```python
from build123d import *

# Parameters (mm, degrees)
F0_W     = 5
F0_H     = 3.3166247904
F0_H_2   = 16
F0_H_3   = 14.6833752096
F0_H_4   = 2
F1_DEPTH = 3
F2_DEPTH = 11
F3_START = 3
F3_DEPTH = 5
F4_R     = 3
F5_F1_R  = 1
F5_F2_R  = 0.9999


# Not quite as in the source:
# - a fillet or chamfer is up to 0.001 mm smaller than in the source, because OpenCascade refuses the exact size


with BuildPart() as f1:
    # F0 (on Top) → F1 (new body)
    with BuildSketch(Plane.XY):
        Rectangle(F0_W, F0_H)
        with Locations((0, -26.3416876048)):
            Rectangle(F0_W, F0_H_2)
        with Locations((0, -11)):
            Rectangle(F0_W, F0_H_3)
        with Locations((0, -2.6583123952)):
            Rectangle(F0_W, F0_H_4)
        Polygon((2.5, -34.3416876048), (-2.5, -34.3416876048), (-2.5, -38.3416876048), (0, -38.3416876048), (2.5, -38.3416876048), align=None)
    extrude(amount=F1_DEPTH)

    # F0 (on Top) → F2 (join)
    with BuildSketch(Plane.XY):
        Rectangle(F0_W, F0_H)
        with Locations((0, -2.6583123952)):
            Rectangle(F0_W, F0_H_4)
        Polygon((2.5, -34.3416876048), (-2.5, -34.3416876048), (-2.5, -38.3416876048), (0, -38.3416876048), (2.5, -38.3416876048), align=None)
        with Locations((0, -26.3416876048)):
            Rectangle(F0_W, F0_H_2)
    extrude(amount=F2_DEPTH)

    # F0 (on Top) → F3 (cut)
    with BuildSketch(Plane.XY.offset(F3_START)):
        with Locations((0, -2.6583123952)):
            Rectangle(F0_W, F0_H_4)
        with Locations((0, -26.3416876048)):
            Rectangle(F0_W, F0_H_2)
    extrude(amount=F3_DEPTH, mode=Mode.SUBTRACT)

    # F4
    f4_edges = [f1.edges().sort_by_distance(p)[0] for p in [
        (0, 1.658312, 11),
        (0, -38.341688, 11),
        (0, -38.341688, 0),
        (0, 1.658312, 0),
    ]]
    fillet(f4_edges, radius=F4_R)

    # F5: fillet of radius 1 on 16 edges, made by hand

    # F5_f1
    f5_f1_edges = [f1.edges().sort_by_distance(p)[0] for p in [
        (0, -34.3416876048, 8),
        (0, -34.3416876048, 3),
        (0, -1.6583123952, 3),
        (0, -1.6583123952, 8),
    ]]
    fillet(f5_f1_edges, radius=F5_F1_R)

    # F5_f2 (radius 1 in the source; OpenCascade refuses exactly that, so slightly less here)
    f5_f2_edges = [f1.edges().sort_by_distance(p)[0] for p in [
        (-2.5, -26.8416876048, 11),
        (2.5, -26.8416876048, 11),
        (2.5, -3.6583123952, 9.5),
        (0, -3.6583123952, 11),
        (-2.5, -3.6583123952, 9.5),
        (0, -3.6583123952, 8),
        (-2.5, -18.3416876048, 9.5),
        (0, -18.3416876048, 11),
        (2.5, -18.3416876048, 9.5),
        (0, -18.3416876048, 8),
        (2.5, -18, 3),
        (-2.5, -18, 3),
        (2.5, -37.4630079484, 10.1213203436),
        (2.5, -38.3416876048, 5.5),
        (2.5, -37.4630079484, 0.8786796564),
        (2.5, -18.3416876048, 0),
        (2.5, 0.7796327387, 0.8786796564),
        (2.5, 1.6583123952, 5.5),
        (2.5, 0.7796327387, 10.1213203436),
        (2.5, -2.5, 11),
        (-2.5, -37.4630079484, 10.1213203436),
        (-2.5, -38.3416876048, 5.5),
        (-2.5, -37.4630079484, 0.8786796564),
        (-2.5, -18.3416876048, 0),
        (-2.5, 0.7796327387, 0.8786796564),
        (-2.5, 1.6583123952, 5.5),
        (-2.5, 0.7796327387, 10.1213203436),
        (-2.5, -2.5, 11),
        (-2.5, -34.048794386, 3.2928932188),
        (-2.5, -1.951205614, 3.2928932188),
        (2.5, -1.951205614, 3.2928932188),
        (2.5, -34.048794386, 3.2928932188),
    ]]
    fillet(f5_f2_edges, radius=F5_F2_R)


solid = f1.part
```
Geometry: final body of the model. Coordinates: model frame, mm. A direction names the side the tool comes from. Round coordinates to 2 decimals unless told otherwise and drop trailing zeros. Write each loop counter-clockwise with the first axis right and the second up, starting at its lowest first coordinate (ties: lowest second). Pieces come first, ordered by that corner, then holes. Notation, with made-up numbers: M 43,-1 L 102,-1 A15 ccw 102,23 Z; hole C 47,33 d1. An arc over 180 degrees is marked long. Answer in a Markdown table with one row per item. Add a question column.
(1) Reachability of faces 1 (the face through (0, -26, 8)), 2 (the face through (-2.215, -17.785, 2.699)), 3 (the face through (2.199, -26.44, 8.285)), 4 (the face through (0.02, -18.63, 10.7)) from +Z, -Z, +X, -X, +Y, -Y: full face, straight path, thin tool, end or side. Return the list, or none.
(2) Cut plane D-D, the plane y = -7. Return the cut outline in (x, z), then the cut area to 3 significant figures.
(3) Ray query, L1, parallel to Z at x = 1.4, y = -21; L2, parallel to Y at x = 1.4, z = 6.5; L3, parallel to Z at x = 0.3, y = -18. Return the intervals inside material, ascending.
(4) Contact query for flat-ended pins moving along their axis: pin 1 (1.5 mm diameter, centred on y = -22, z = 5, fed in from -X); pin 2 (1.1 mm diameter, centred on x = 0.5, z = 9.5, fed in from -Y). Output: stop coordinate, or through.
(5) Cut plane A-A, the plane z = 6.5. Return the cut outline in (x, y), then the cut area to 3 significant figures.
(6) Draft query along Y for faces 5 (the face through (0, -38.342, 5)), 6 (the face through (-2.21, -1.36, 5.52)), 7 (the face through (0, 1.658, 5)). Return one class per face: pulls with the +Y half, pulls with the -Y half, needs draft (parallel to the pull), parting line crosses it, or undercut.
(7) Cut plane B-B, the plane y = -23. Return the cut outline in (x, z).
Established:
| question | item | result |
|---|---|---|
| 1 | face 1 | +X, -X |
| 1 | face 2 | -X |
| 1 | face 3 | +X |
| 1 | face 4 | +Z, +X, -X |
| 2 | outline | M -2.5,1 A1 ccw -1.5,0 L 1.5,0 A1 ccw 2.5,1 L 2.5,2 A1 ccw 1.5,3 L -1.5,3 A1 ccw -2.5,2 Z |
| 2 | area | 14.1 mm² |
| 3 | L1 | 0 to 3, 8 to 11 |
| 3 | L2 | -38.34 to -34.34, -1.66 to 1.66 |
| 3 | L3 | 0 to 3 |
| 4 | pin 1 | through |
| 4 | pin 2 | y = -38.19 |
| 5 | outline | M -2.5,-37.34 A1 ccw -1.5,-38.34 L 1.5,-38.34 A1 ccw 2.5,-37.34 L 2.5,-35.34 A1 ccw 1.5,-34.34 L -1.5,-34.34 A1 ccw -2.5,-35.34 Z; M -2.5,-0.66 A1 ccw -1.5,-1.66 L 1.5,-1.66 A1 ccw 2.5,-0.66 L 2.5,0.66 A1 ccw 1.5,1.66 L -1.5,1.66 A1 ccw -2.5,0.66 Z |
| 5 | area | 34.9 mm² |
| 6 | face 5 | pulls with the -Y half |
| 6 | face 6 | undercut |
| 6 | face 7 | pulls with the +Y half |
| 7 | outline | M -2.5,1 A1 ccw -1.5,0 L 1.5,0 A1 ccw 2.5,1 L 2.5,2 A1 ccw 1.5,3 L -1.5,3 A1 ccw -2.5,2 Z; M -2.5,9 A1 ccw -1.5,8 L 1.5,8 A1 ccw 2.5,9 L 2.5,10 A1 ccw 1.5,11 L -1.5,11 A1 ccw -2.5,10 Z |
